Geometry: see drawing. Coordinates: mm, zero at the bounding-box minimum. A direction names the side the tool comes from. Give positions to 0.01 mm unless a question says otherwise; leave off trailing zeros. Order: outer loops, then holes, each group sorted by start corner. A loop starts at its lowest first (then second) coordinate and runs counter-clockwise, first axis right, second up. Notation, with made-up numbers: M -18.5,62.25 L 0.5,62.25 A16 cw 0.5,88.25 Z; hole C -9,-2.75 d9. An arc over 180 degrees is marked long. Return JSON: item names as keys, results as strings.
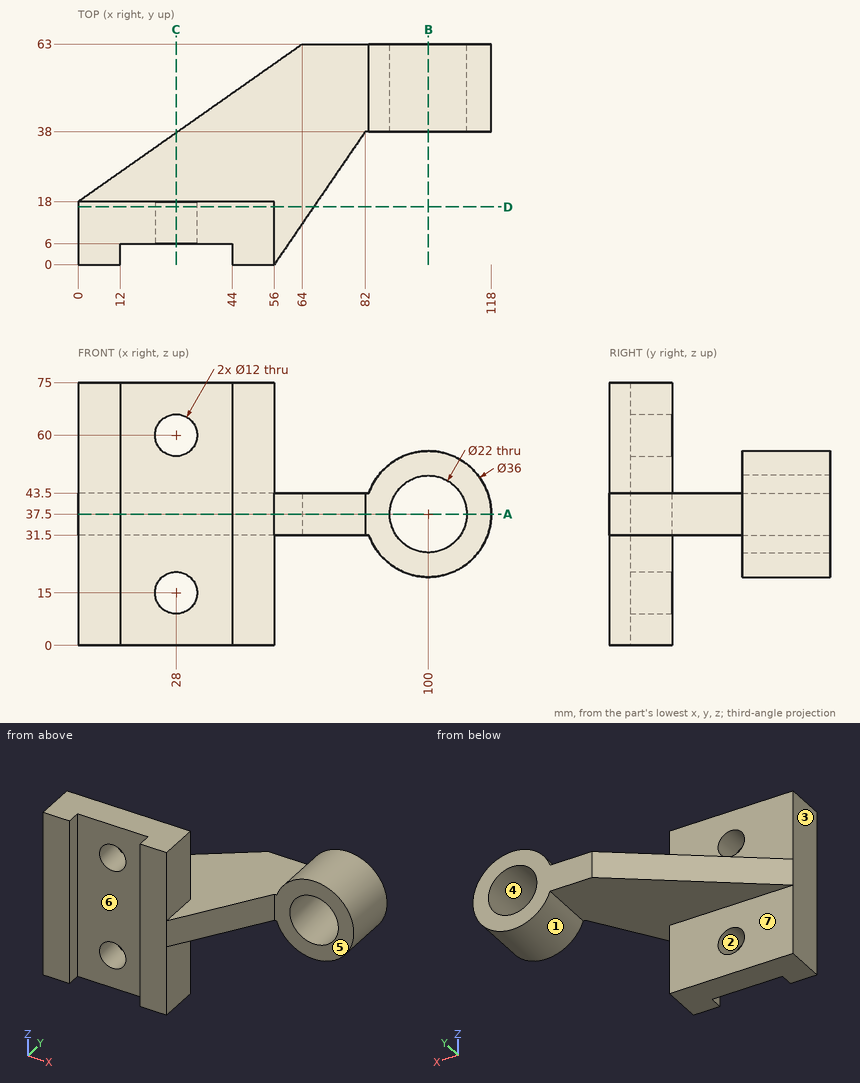
1. Section query B-B (x = 100). Return loops of the section in (y, z), then the cut area to 3 significant figures.
Evaluation:
{"outline": "M 38,19.5 L 63,19.5 L 63,26.5 L 38,26.5 Z; M 38,48.5 L 63,48.5 L 63,55.5 L 38,55.5 Z", "area": "350 mm^2"}
2. Ray query, probe 1 along Z at (x, y) = (28, 14); probe 2 along Z at (x, y) = (27, 17); probe 3 along X at (y, z) = (13.5, 13). Return the intervals inside material, ascending.
Evaluation:
{"probe 1": "z = 0 to 9, 21 to 54, 66 to 75", "probe 2": "z = 0 to 9.08, 20.92 to 54.08, 65.92 to 75", "probe 3": "x = 0 to 22.34, 33.66 to 56"}
3. Set-up query: the marked faces 5, 6 and 7. Return all of +Z, -Z, +X, -X, +Y, -Y with unobstructed straight access to the full face (end or side cutting, diameter ignored); none if empty.
Evaluation:
{"face 5": "+Z, -Z, +X, -Y", "face 6": "+Z, -Z, -Y", "face 7": "-Z, +X, -X, +Y"}
4. Section query C-C (x = 28). Return loops of the section in (y, z).
Evaluation:
{"outline": "M 6,0 L 18,0 L 18,9 L 6,9 Z; M 6,21 L 18,21 L 18,31.5 L 37.69,31.5 L 37.69,43.5 L 18,43.5 L 18,54 L 6,54 Z; M 6,66 L 18,66 L 18,75 L 6,75 Z"}
5. First-contact query: pin 1 (1.8 mm diameter, centred on y = 2, z = 26.5, fed in from +X); pin 2 (1 mm diameter, centred on x = 40, z = 27, fed in from +Y); pin 3 (11 mm diameter, centred on x = 28, z = 15, fed in from +Y); pin 4 (19 mm diameter, centred on x = 24, y = 35, fed in from +Z). Flat tips, straight axial feed; report the tip coordinate or a pass-through.
Evaluation:
{"pin 1": "stops at x = 56", "pin 2": "stops at y = 18", "pin 3": "passes through", "pin 4": "stops at z = 43.5"}
6. Section query A-A (z = 37.5). Return loops of the section in (x, y).
Evaluation:
{"outline": "M 0,0 L 12,0 L 12,6 L 44,6 L 44,0 L 56,0 L 82,38 L 89,38 L 89,63 L 64,63 L 0,18 Z; M 111,38 L 118,38 L 118,63 L 111,63 Z"}
7. Section query D-D (y = 16.5). Return loops of the section in (x, z), then the cut area to 3 significant figures.
Evaluation:
{"outline": "M 0,0 L 56,0 L 56,31.5 L 67.29,31.5 L 67.29,43.5 L 56,43.5 L 56,75 L 0,75 Z; hole C 28,15 d12; hole C 28,60 d12", "area": "4,110 mm^2"}
8. Draft query along Z for the marked faces 1, 2, 3 and 4. Return one class per face: pulls with the +Z half, pulls with the -Z half, needs draft (parallel to the pull), parting line crosses it, or undercut.
Evaluation:
{"face 1": "parting line crosses it", "face 2": "undercut", "face 3": "needs draft", "face 4": "undercut"}
